Autodesk Inventor part; units mm, degrees
ref_plane "YZ Plane" through (0, 0, 0) normal (1, 0, 0) x (0, 1, 0)
ref_plane "XZ Plane" through (0, 0, 0) normal (0, 1, 0) x (-1, 0, 0)
ref_plane "XY Plane" through (0, 0, 0) normal (0, 0, 1) x (1, 0, 0)
sketch "Sketch4" plane through (0, 0, 0) normal (1, 0, 0) x (0, 1, 0)
  line L0 (88.8188, -396.6218) -> (88.8188, -1896.6218)
  line L1 (88.8188, -1896.6218) -> (238.8188, -1896.6218)
  line L2 (238.8188, -1896.6218) -> (238.8188, -1821.6218)
  line L3 (238.8188, -1821.6218) -> (367.6368, -1694.6481)
  line L4 (367.6368, -1694.6481) -> (367.6368, -1494.6481)
  line L5 (367.6368, -1494.6481) -> (238.8188, -1401.7722)
  line L6 (238.8188, -1401.7722) -> (238.8188, -1326.7722)
  line L7 (238.8188, -1326.7722) -> (367.6368, -1148.1032)
  line L8 (367.6368, -1148.1032) -> (367.6368, -948.1032)
  line L9 (367.6368, -948.1032) -> (238.8188, -817.4142)
  line L10 (238.8188, -817.4142) -> (238.8188, -742.4142)
  line L11 (238.8188, -742.4142) -> (367.6368, -615.4405)
  line L12 (367.6368, -615.4405) -> (367.6368, -415.4405)
  line L13 (367.6368, -415.4405) -> (238.8188, -284.7516)
  line L14 (238.8188, -284.7516) -> (88.8188, -284.7516)
  line L15 (88.8188, -284.7516) -> (88.8188, -396.6218)
  point P0 (0, 0)
  dimension "d47" = 1500
  dimension "d48" = 150
  dimension "d49" = 75
  dimension "d50" = 200
  dimension "d51" = 75
  dimension "d52" = 200
  dimension "d53" = 75
  dimension "d54" = 200
extrude "Extrusion4" add sketch "Sketch4" along normal blind 400
fillet "Fillet5" radius 50 12 edges at (200, 367.6368, -415.4405) (400, 367.6368, -515.4405) (200, 367.6368, -615.4405) (200, 367.6368, -948.1032) (0, 367.6368, -515.4405) (0, 367.6368, -1048.1032) (200, 367.6368, -1148.1032) (400, 367.6368, -1048.1032) (200, 367.6368, -1494.6481) (400, 367.6368, -1594.6481) (200, 367.6368, -1694.6481) (0, 367.6368, -1594.6481)
properties part number "mould"
For this review, take the finished solid that the model builds, in its own axes (mm). A direction names the side the tool comes from. Round coordinates to 2 decimals unless told otherwise and drop trailing zeros. Write each loop counter-clockwise with the first axis right and the second up, starting at its lowest first coordinate (ties: lowest second). Pieces come first, ordered by that corner, then holes. Notation, with made-up numbers: M 7,-28.75 L 27,-28.75 A10 ccw 27,-12.75 Z; hole C 31,25 d1. An arc over 180 degrees is marked long. Write item = value, one per line. Start each with the question number.
(1) For faces 1 (the face through (197.2, 297.671, -1245.145)), 2 (the face through (202.599, 363.654, -1693.282)), list the 3-axis set-ups (+Z, -Z, +X, -X, +Y, -Y) from which the entire face can be reached by the end or side of a thin tool; tool diameter is ignored.
(2) We need section B-B (x = 220). Give the boundary of the cut face in (y, z).
(3) We need section A-A (y = 287). Give the boundary of the cut face in (x, z), then the cut area to 3 significant figures.
(4) Clearance check with flat-ended pins moving along their axes: pin 1 Ø1.5 at (x, z) = (79.5, -650) entering from +Y; pin 2 Ø1.5 at (x, z) = (69.5, -1473.5) entering from +Y; pin 3 Ø10 at (x, y) = (91.5, 260.5) entering from +Z. State where each tip first meets the part, or that it passes through.
(5) We need section C-C (z = -417.5). Give the boundary of the cut face in (x, y), then the cut area to 3 significant figures.
(6) For line 1 along Z through (x, y) = (71.5, 285); line 2 along Z through (x, y) = (200.5, 333); line 3 along Y through (x, z) = (334, -824.5), list the stretches that pass through material, from the lowest coordinate up.
(7) We need section D-D (z = -1378.5). Give the boundary of the cut face in (x, y), then the cut area to 3 significant figures.
(8) The part is to be moulded in two halves that separate along Z. For faces 3 (the face through (391.27, 345.864, -512.619)), 4 (the face through (197.2, 296.833, -343.609)), 5 (the face through (202.599, 363.654, -614.075)), say which applies: +Z half, -Z half, draft (parallel to the pull), parting line (faces both ways), or undercut.
Results found:
q1.face_1 = +X, -X, +Y
q1.face_2 = -Z, +X, -X, +Y
q2.outline = M 88.82,-1896.62 L 238.82,-1896.62 L 238.82,-1821.62 L 352.74,-1709.34 A50 ccw 367.64,-1673.73 L 367.64,-1520.24 A50 ccw 346.88,-1479.68 L 238.82,-1401.77 L 238.82,-1326.77 L 358.19,-1161.2 A50 ccw 367.64,-1131.96 L 367.64,-968.6 A50 ccw 353.25,-933.5 L 238.82,-817.41 L 238.82,-742.41 L 352.74,-630.13 A50 ccw 367.64,-594.52 L 367.64,-435.94 A50 ccw 353.25,-400.84 L 238.82,-284.75 L 88.82,-284.75 Z
q3.outline = M 0,-1774.13 L 400,-1774.13 L 400,-1436.51 L 0,-1436.51 Z; M 0,-1259.95 L 400,-1259.95 L 400,-866.3 L 0,-866.3 Z; M 0,-694.92 L 400,-694.92 L 400,-333.63 L 0,-333.63 Z
q3.area = 437,000 mm²
q4.pin_1 = 333.34
q4.pin_2 = 339.34
q4.pin_3 = -301.68
q5.outline = M 0,88.82 L 400,88.82 L 400,317.64 A50 ccw 368.44,364.11 L 31.56,364.11 A50 ccw 0,317.64 Z
q5.area = 109,000 mm²
q6.line_1 = -1776.1 to -1435.07, -1262.72 to -864.27, -696.89 to -331.6
q6.line_2 = -1728.79 to -1469.68, -1196.14 to -912.96, -649.58 to -380.3
q6.line_3 = 88.82 to 245.8
q7.outline = M 0,88.82 L 400,88.82 L 400,238.82 L 0,238.82 Z
q7.area = 60,000 mm²
q8.face_3 = draft
q8.face_4 = +Z half
q8.face_5 = undercut
